```python
from build123d import *

# Parameters (mm, degrees)
BOSS_EXTRUDE1_DEPTH = 2.2
SKETCH2_R           = 19.45
BOSS_EXTRUDE2_DEPTH = 7
CHAMFER1_SIZE       = 0.75


with BuildPart() as part:
    # Sketch1 → Boss-Extrude1 (new body)
    with BuildSketch(Plane(origin=(0, 0, 0), x_dir=(1, 0, 0), z_dir=(0, 1, 0))):
        with BuildLine():
            Line((-8.25, 19.854155736), (-8.25, 33.5))
            Line((-8.25, 33.5), (8.25, 33.5))
            Line((8.25, 33.5), (8.25, 19.854155736))
            ThreePointArc((8.25, 19.854155736), (0, -21.5), (-8.25, 19.854155736))
        make_face()
    extrude(amount=BOSS_EXTRUDE1_DEPTH)

    # Sketch2 → Boss-Extrude2 (add)
    with BuildSketch(Plane(origin=(0, 2.2, 0), x_dir=(1, 0, 0), z_dir=(0, 1, 0))):
        with Locations(Location((0, 0, 0), (0, 0, 270))):
            Circle(SKETCH2_R)
    extrude(amount=BOSS_EXTRUDE2_DEPTH)

    # Chamfer1
    chamfer1_edges = [part.edges().sort_by_distance(p)[0] for p in [
        (0, 2.2, -33.5),
        (0, 9.2, -19.45),
        (-8.25, 2.2, -26.677077868),
        (0, 2.2, 21.5),
        (-8.25, 0, -26.677077868),
        (0, 0, -33.5),
        (8.25, 0, -26.677077868),
        (0, 0, 21.5),
        (8.25, 2.2, -26.677077868),
    ]]
    chamfer(chamfer1_edges, length=CHAMFER1_SIZE)


solid = part.part
```
Build history of the part. All positions in model axes, mm. A direction names the side the tool comes from. Round coordinates to 2 decimals unless told otherwise and drop trailing zeros. Order: outer loops, then holes, each group sorted by start corner. A loop starts at its lowest first (then second) coordinate and runs counter-clockwise, first axis right, second up. Notation, with made-up numbers: (60, 0.5) -> (65, 0.5) arc R21 ccw to (65, 39.5) -> close; hole circle Ø1 at (83, 60). An arc over 180 degrees is marked (long way). Answer in a Markdown table with one row per item.
1) Band-saw the part on A-A on z = 0. Give the cut face in (x, y), and give its area (3 significant figures).
Values:
| item | result |
|---|---|
| outline | (-21.5, 0.75) -> (-20.75, 0) -> (20.75, 0) -> (21.5, 0.75) -> (21.5, 1.45) -> (20.75, 2.2) -> (19.45, 2.2) -> (19.45, 8.45) -> (18.7, 9.2) -> (-18.7, 9.2) -> (-19.45, 8.45) -> (-19.45, 2.2) -> (-20.75, 2.2) -> (-21.5, 1.45) -> close |
| area | 365 mm2 |
2) Band-saw the part on D-D on z = -27.5. Give the cut face in (x, y), and give its area (3 significant figures).
Values:
| item | result |
|---|---|
| outline | (-8.25, 0.75) -> (-7.5, 0) -> (7.5, 0) -> (8.25, 0.75) -> (8.25, 1.45) -> (7.5, 2.2) -> (-7.5, 2.2) -> (-8.25, 1.45) -> close |
| area | 35.2 mm2 |
3) Band-saw the part on B-B on x = 0. Give the cut face in (y, z).
Values:
| item | result |
|---|---|
| outline | (0, -32.75) -> (0.75, -33.5) -> (1.45, -33.5) -> (2.2, -32.75) -> (2.2, -19.45) -> (8.45, -19.45) -> (9.2, -18.7) -> (9.2, 18.7) -> (8.45, 19.45) -> (2.2, 19.45) -> (2.2, 20.75) -> (1.45, 21.5) -> (0.75, 21.5) -> (0, 20.75) -> close |
4) Band-saw the part on C-C on y = 4.5. Give the cut face in (x, z), and give its area (3 significant figures).
Values:
| item | result |
|---|---|
| outline | circle Ø38.9 at (0, 0) |
| area | 1,190 mm2 |
5) Which spindle directions (+Z, -Z, +X, -X, +Y, -Y) get a long thin tool onto all of the face, cutting with end or side? Do faces 1 (the flat face through (0, 2.2, -20)), 2 (the conical face through (0.81, 0.12, 20.854)). Say none if no direction does.
Values:
| item | result |
|---|---|
| face 1 | +Y |
| face 2 | -Y |
6) Pin check, flat tips, straight feed: P1, Ø5, axis at y = 1, z = 15, coming from the +X side; P2, Ø1.5, axis at y = 6, z = -2, coming from the -X side. Stop position of each tip, or through.
Values:
| item | result |
|---|---|
| P1 | x = 17.49 |
| P2 | x = -19.41 |
7) Wall check: L1, parallel to Y at x = 18, z = 9; L2, parallel to X at y = 6, z = -16; L3, parallel to X at y = 8.5, z = -15.5. Give the ranges that are in metal, low to high.
Values:
| item | result |
|---|---|
| L1 | 0 to 2.2 |
| L2 | -11.06 to 11.06 |
| L3 | -11.67 to 11.67 |
